Verification items for the finished model (mm, model axes). Face numbers are marked on the shaded views. A direction names the side the tool comes from. Give positions to 0.01 mm unless a question says otherwise; leave off trailing zeros. Answer as a JSON object with one key per item and string values.
```python
from build123d import *

# Parameters (mm, degrees)
SKETCH1_W           = 127.7
SKETCH1_H           = 85.9
BOSS_EXTRUDE1_DEPTH = 28.1
SKETCH2_R           = 13.9
CUT_EXTRUDE3_DEPTH  = 25
CHAMFER3_SIZE       = 1
CHAMFER4_SIZE       = 1
SKETCH3_R           = 13.9
CUT_EXTRUDE5_DEPTH  = 25
CHAMFER5_SIZE       = 1
CHAMFER6_SIZE       = 1
SKETCH5_R           = 2
CUT_EXTRUDE7_DEPTH  = 10


with BuildPart() as part:
    # Sketch1 → Boss-Extrude1 (new body)
    with BuildSketch(Plane(origin=(0, 0, 0), x_dir=(1, 0, 0), z_dir=(0, 1, 0))):
        with Locations((-248.856003869, 89.066665881)):
            Rectangle(SKETCH1_W, SKETCH1_H)
    extrude(amount=BOSS_EXTRUDE1_DEPTH)

    # Sketch2 → Cut-Extrude3 (cut)
    with BuildSketch(Plane(origin=(0, 0, 0), x_dir=(-1, 0, 0), z_dir=(0, -1, 0))):
        with Locations((294.706003869, 64.116665881)):
            Circle(SKETCH2_R)
        with Locations((264.136003869, 64.116665881)):
            Circle(SKETCH2_R)
        with Locations((233.566003869, 64.116665881)):
            Circle(SKETCH2_R)
        with Locations((203.006003869, 64.116665881)):
            Circle(SKETCH2_R)
    extrude(amount=-CUT_EXTRUDE3_DEPTH, mode=Mode.SUBTRACT)

    # Chamfer3
    chamfer3_edges = [part.edges().sort_by_distance(p)[0] for p in [
        (-250.236003869, 0, -64.116665881),
    ]]
    chamfer(chamfer3_edges, length=CHAMFER3_SIZE)

    # Chamfer4
    chamfer4_edges = [part.edges().sort_by_distance(p)[0] for p in [
        (-280.806003869, 0, -64.116665881),
        (-189.106003869, 0, -64.116665881),
        (-219.666003869, 0, -64.116665881),
    ]]
    chamfer(chamfer4_edges, length=CHAMFER4_SIZE)

    # Sketch3 → Cut-Extrude5 (cut)
    with BuildSketch(Plane.XZ):
        with Locations((-233.566003869, -114.016665881)):
            Circle(SKETCH3_R)
        with Locations((-264.136003869, -114.016665881)):
            Circle(SKETCH3_R)
        with Locations((-294.706003869, -114.016665881)):
            Circle(SKETCH3_R)
        with Locations((-203.006003869, -114.016665881)):
            Circle(SKETCH3_R)
    extrude(amount=-CUT_EXTRUDE5_DEPTH, mode=Mode.SUBTRACT)

    # Chamfer5
    chamfer5_edges = [part.edges().sort_by_distance(p)[0] for p in [
        (-308.606003869, 0, -114.016665881),
        (-278.036003869, 0, -114.016665881),
        (-216.906003869, 0, -114.016665881),
        (-247.466003869, 0, -114.016665881),
    ]]
    chamfer(chamfer5_edges, length=CHAMFER5_SIZE)

    # Chamfer6
    chamfer6_edges = [part.edges().sort_by_distance(p)[0] for p in [
        (-248.856003869, 0, -132.016665881),
        (-185.006003869, 0, -89.066665881),
        (-248.856003869, 0, -46.116665881),
        (-312.706003869, 0, -89.066665881),
    ]]
    chamfer(chamfer6_edges, length=CHAMFER6_SIZE)

    # Sketch5 → Cut-Extrude7 (cut)
    with BuildSketch(Plane(origin=(0, 25, 0), x_dir=(-1, 0, 0), z_dir=(0, -1, 0))):
        with Locations((294.706003869, 64.116665881)):
            Circle(SKETCH5_R)
        with Locations((264.136003869, 64.116665881)):
            Circle(SKETCH5_R)
        with Locations((233.566003869, 64.116665881)):
            Circle(SKETCH5_R)
        with Locations((203.006003869, 64.116665881)):
            Circle(SKETCH5_R)
        with Locations((294.706003869, 114.016665881)):
            Circle(SKETCH5_R)
        with Locations((264.136003869, 114.016665881)):
            Circle(SKETCH5_R)
        with Locations((233.566003869, 114.016665881)):
            Circle(SKETCH5_R)
        with Locations((203.006003869, 114.016665881)):
            Circle(SKETCH5_R)
    extrude(amount=-CUT_EXTRUDE7_DEPTH, mode=Mode.SUBTRACT)


solid = part.part
```
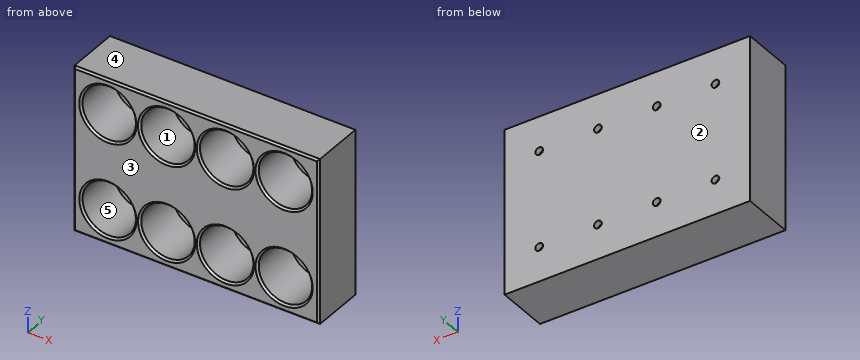
Q1. Release check for a two-part mould opening along Z. For the marked faces 3, 4 and 5 record: +Z half, -Z half, draft (parallel to the pull), parting line (faces both ways), or undercut.
Resolved:
{"face 3": "draft", "face 4": "+Z half", "face 5": "undercut"}
Q2. Section check A-A on y = 16. Count the separate pieces of the cut face and the enclosed holes in it, then the cut area to 3 significant figures.
Resolved:
{"separate pieces": "1", "enclosed holes": "8", "area": "6,110 mm²"}
Q3. Gauge pin test, flat end, axial feed: pin 1 Ø6.5 at (x, z) = (-264.14, -64.12) entering from -Y. Record the tip position at first contact, or that the pin passes through.
Resolved:
{"pin 1": "stops at y = 25"}
Q4. Tool access check on the marked faces 1 and 2. Record the directions out of +Z, -Z, +X, -X, +Y, -Y that give a thin tool (end or side, any length) a straight path to the whole face; none if there is none.
Resolved:
{"face 1": "-Y", "face 2": "+Z, -Z, +X, -X, +Y"}
Q5. Material ranges on L1, parallel to X at y = 3.25, z = -114; L2, parallel to X at y = 3.5, z = -53.5; L3, parallel to Z at x = -291, y = 18, recorded low to high.
Resolved:
{"L1": "x = -312.71 to -308.61, -280.81 to -278.04, -250.24 to -247.47, -219.67 to -216.91, -189.11 to -185.01", "L2": "x = -312.71 to -303.68, -285.73 to -273.11, -255.16 to -242.54, -224.59 to -211.98, -194.03 to -185.01", "L3": "z = -132.02 to -127.41, -100.62 to -77.51, -50.72 to -46.12"}
